Could you check a few things on this model? Use its own coordinates, in mm. A direction names the side the tool comes from. Give positions to 0.01 mm unless a question says otherwise; leave off trailing zeros. Order: outer loops, then holes, each group sorted by start corner. A loop starts at its lowest first (then second) coordinate and runs counter-clockwise, first axis right, second up.
from build123d import *

# Parameters (mm, degrees)
EXTRUDE1_DEPTH  = 100
SKETCH2_R       = 3
EXTRUDE2_DEPTH  = 3.5
SKETCH_R        = 1.75
EXTRUDE3_DEPTH  = 7.5
LPATTERN1_COUNT = 13
LPATTERN1_PITCH = 20


with BuildPart() as part:
    # Sketch1 → Extrude1 (new body)
    with BuildSketch(Plane.XY):
        with BuildLine():
            Line((-4.5, -3.25), (4.5, -3.25))
            Line((4.5, -3.25), (4.5, 0.25))
            ThreePointArc((4.5, 0.25), (3.93077967, 0.427814974), (3.563991137, 0.898023568))
            Line((3.563991137, 0.898023568), (3.235073025, 0.898023568))
            Line((3.235073025, 0.898023568), (3.235073025, 1.601976432))
            Line((3.235073025, 1.601976432), (3.563991137, 1.601976432))
            ThreePointArc((3.563991137, 1.601976432), (3.93077967, 2.072185026), (4.5, 2.25))
            Line((4.5, 2.25), (4.5, 3.25))
            Line((4.5, 3.25), (-4.5, 3.25))
            Line((-4.5, 3.25), (-4.5, 2.25))
            ThreePointArc((-4.5, 2.25), (-3.93077967, 2.072185026), (-3.563991137, 1.601976432))
            Line((-3.563991137, 1.601976432), (-3.235073025, 1.601976432))
            Line((-3.235073025, 1.601976432), (-3.235073025, 0.898023568))
            Line((-3.235073025, 0.898023568), (-3.563991137, 0.898023568))
            ThreePointArc((-3.563991137, 0.898023568), (-3.93077967, 0.427814974), (-4.5, 0.25))
            Line((-4.5, 0.25), (-4.5, -3.25))
        make_face()
    extrude(amount=EXTRUDE1_DEPTH)

    # Sketch2 → Extrude2 (cut)
    with BuildSketch(Plane(origin=(0, 3.25, 0), x_dir=(1, 0, 0), z_dir=(0, 1, 0))):
        with Locations((0, -10)):
            Circle(SKETCH2_R)
    extrude2 = extrude(amount=-EXTRUDE2_DEPTH, mode=Mode.SUBTRACT)

    # Sketch → Extrude3 (cut, through all)
    with BuildSketch(Plane(origin=(0, 3.25, 0), x_dir=(1, 0, 0), z_dir=(0, 1, 0))):
        with Locations((0, -10)):
            Circle(SKETCH_R)
    extrude3 = extrude(amount=-EXTRUDE3_DEPTH, mode=Mode.SUBTRACT)

    # LPattern1: Extrude2, Extrude3 ×13
    with Locations(*[(0, 0, i * LPATTERN1_PITCH) for i in range(1, LPATTERN1_COUNT)]):
        add(extrude2, mode=Mode.SUBTRACT)
        add(extrude3, mode=Mode.SUBTRACT)


solid = part.part
Item 1: Imagine slicing it at A-A on z = 90. List the corners of the cut face in (x, y) for me.
Findings:
outline: (-4.5, -3.25) - (-1.75, -3.25) - (-1.75, -0.25) - (-3, -0.25) - (-3, 3.25) - (-4.5, 3.25) - (-4.5, 2.25) arc R1 cw to (-3.56, 1.6) - (-3.24, 1.6) - (-3.24, 0.9) - (-3.56, 0.9) arc R1 cw to (-4.5, 0.25) - close; (1.75, -3.25) - (4.5, -3.25) - (4.5, 0.25) arc R1 cw to (3.56, 0.9) - (3.24, 0.9) - (3.24, 1.6) - (3.56, 1.6) arc R1 cw to (4.5, 2.25) - (4.5, 3.25) - (3, 3.25) - (3, -0.25) - (1.75, -0.25) - close
Item 2: For faces 5 (the flat face through (0, -0.25, 12)), 6 (the cylindrical face through (-0.38, -1.73, 51.71)), which set-ups out of +Z, -Z, +X, -X, +Y, -Y let a thin tool reach every point of the face, with its end or its side?
Findings:
face 5: +Y
face 6: +Y, -Y
Item 3: Imagine slicing it at B-B on z = 14. List the corners of the cut face in (x, y) for me.
Findings:
outline: (-4.5, -3.25) - (4.5, -3.25) - (4.5, 0.25) arc R1 cw to (3.56, 0.9) - (3.24, 0.9) - (3.24, 1.6) - (3.56, 1.6) arc R1 cw to (4.5, 2.25) - (4.5, 3.25) - (-4.5, 3.25) - (-4.5, 2.25) arc R1 cw to (-3.56, 1.6) - (-3.24, 1.6) - (-3.24, 0.9) - (-3.56, 0.9) arc R1 cw to (-4.5, 0.25) - close
Item 4: Imagine slicing it at C-C on x = 0. Give the number of separate pieces and of enclosed holes in the cut face, then the cut area to 4 significant figures.
Findings:
separate pieces: 6
enclosed holes: 0
area: 492.5 mm2
Item 5: For pin 1 (0.6 mm diameter, centred on y = 1.5, z = 47, fed in from +X); pin 2 (1.8 mm diameter, centred on x = 0.5, z = 31, fed in from +Y); pin 3 (1 mm diameter, centred on y = 1.5, z = 51, fed in from -X), each with a flat end and sliding along its axis, tell me the tip position at first contact or that it passes through.
Findings:
pin 1: stops at x = 3.66
pin 2: stops at y = -0.25
pin 3: stops at x = -3.84
Item 6: We'd pull the mould along X, two halves only. Please class faces 1 (the flat face through (3, 3.25, 49)), 2 (the flat face through (4.5, -2, 49)), 3 (the flat face through (-4.5, -1, 49)), 4 (the flat face through (2, -0.25, 70)): +X half, -X half, draft (parallel to the pull), parting line (faces both ways), or undercut.
Findings:
face 1: draft
face 2: +X half
face 3: -X half
face 4: undercut
Item 7: Please list where these lines run through material, in increasing order: line 1 along X through (y, z) = (-0.95, 70); line 2 along X through (y, z) = (0, 90); line 3 along Z through (x, y) = (0, -2).
Findings:
line 1: x = -4.5 to -1.75, 1.75 to 4.5
line 2: x = -4.5 to -3, 3 to 4.5
line 3: z = 0 to 8.25, 11.75 to 28.25, 31.75 to 48.25, 51.75 to 68.25, 71.75 to 88.25, 91.75 to 100
